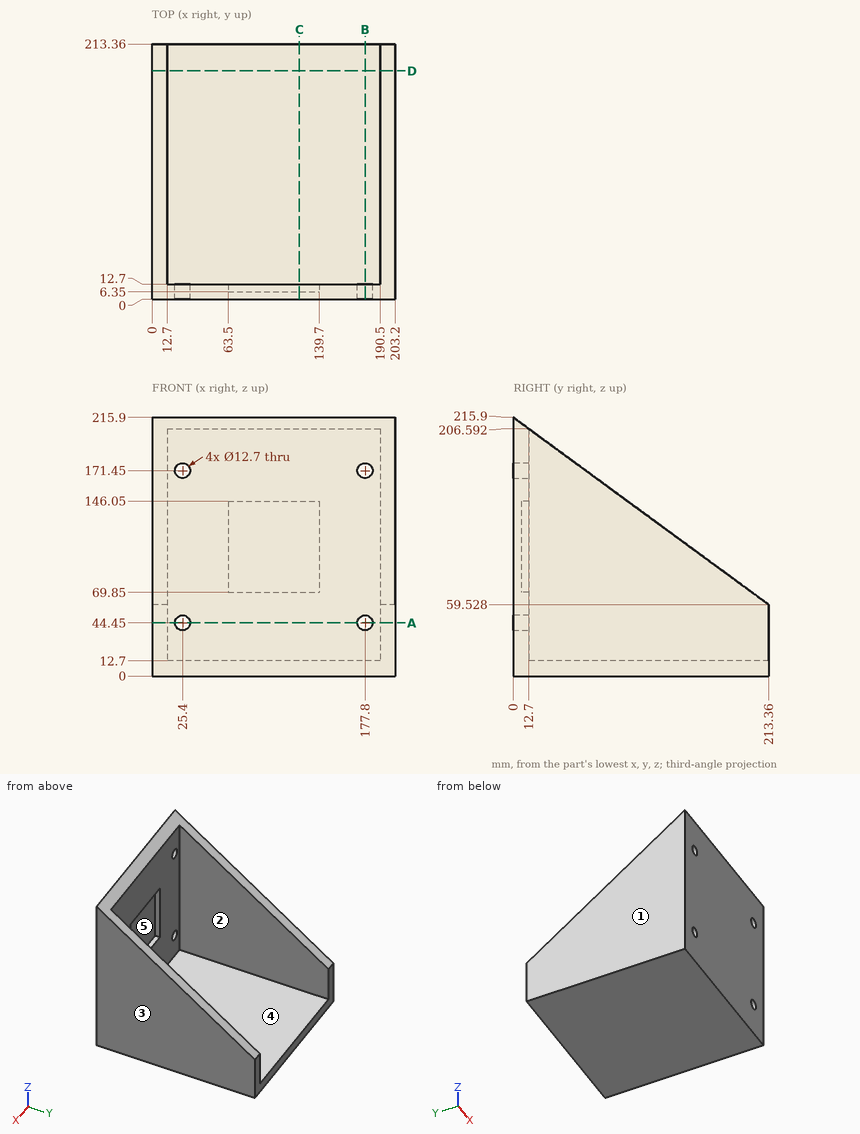
Print and shaded views of the part. All mm, measured from the part's lowest x, y and z. A direction names the side the tool comes from. Give positions to 0.01 mm unless a question says otherwise; leave off trailing zeros. Loops run counter-clockwise (first coordinate to the right, second up) from the corner with the lowest first, then second, coordinate; pieces in that order, holes last. Notation, with made-up numbers: (62.5, 0.25) -> (84.5, 0.25) arc R12 cw to (84.5, 14.25) -> close; hole circle Ø7 at (23.25, 58). An arc over 180 degrees is marked (long way). Use CSV: the item, a comma, the result in double quotes. Start each with the question number.
1) Mould opens along Z. For the marked faces 3, 4 and 5 say: released by +Z, released by -Z, zero draft, split by the parting line, or undercut.
2) Slice it at D-D on y = 191. Give the cut face in (x, z), plus the area to 3 significant figures.
3) Flat gauge pins, fed straight in: pin 1 Ø20.5 at (x, z) = (25.4, 171.45) entering from +Y; pin 2 Ø5 at (x, y) = (164.5, 72) entering from +Z; pin 3 Ø5 at (x, y) = (102.5, 8.5) entering from +Z. Where does each tip first touch, or does it go through?
4) Slice it at B-B on x = 177.8. Give the cut face in (y, z), plus the area to 3 significant figures.
5) Slice it at C-C on x = 123. Give the cut face in (y, z).
6) Wall check: line 1 (X direction, y = 7, z = 44.45); line 2 (X direction, y = 157, z = 58.5); line 3 (Z direction, x = 177.8, y = 6.5). Give the ranges that are in metal, low to high.
7) Slice it at A-A on z = 44.45. Give the cut face in (x, y).
8) Tool access for the marked faces 1 and 2: list every direction of +Z, -Z, +X, -X, +Y, -Y with a clear straight run to the whole face (end or side of a thin tool).
Computed values:
1,face 3,"zero draft"
1,face 4,"released by +Z"
1,face 5,"undercut"
2,outline,"(0, 0) -> (203.2, 0) -> (203.2, 75.92) -> (190.5, 75.92) -> (190.5, 12.7) -> (12.7, 12.7) -> (12.7, 75.92) -> (0, 75.92) -> close"
2,area,"4,190 mm^2"
3,pin 1,"stops at y = 12.7"
3,pin 2,"stops at z = 12.7"
3,pin 3,"stops at z = 211.5"
4,outline,"(0, 0) -> (213.36, 0) -> (213.36, 12.7) -> (12.7, 12.7) -> (12.7, 38.1) -> (0, 38.1) -> close; (0, 50.8) -> (12.7, 50.8) -> (12.7, 165.1) -> (0, 165.1) -> close; (0, 177.8) -> (12.7, 177.8) -> (12.7, 206.59) -> (0, 215.9) -> close"
4,area,"4,910 mm^2"
5,outline,"(0, 0) -> (213.36, 0) -> (213.36, 12.7) -> (12.7, 12.7) -> (12.7, 69.85) -> (6.35, 69.85) -> (6.35, 146.05) -> (12.7, 146.05) -> (12.7, 206.59) -> (0, 215.9) -> close"
6,line 1,"x = 0 to 19.05, 31.75 to 171.45, 184.15 to 203.2"
6,line 2,"x = 0 to 12.7, 190.5 to 203.2"
6,line 3,"z = 0 to 38.1, 50.8 to 165.1, 177.8 to 211.14"
7,outline,"(0, 0) -> (19.05, 0) -> (19.05, 12.7) -> (12.7, 12.7) -> (12.7, 213.36) -> (0, 213.36) -> close; (31.75, 0) -> (171.45, 0) -> (171.45, 12.7) -> (31.75, 12.7) -> close; (184.15, 0) -> (203.2, 0) -> (203.2, 213.36) -> (190.5, 213.36) -> (190.5, 12.7) -> (184.15, 12.7) -> close"
8,face 1,"+Z, -Z, -X, +Y, -Y"
8,face 2,"+Z, +Y"
